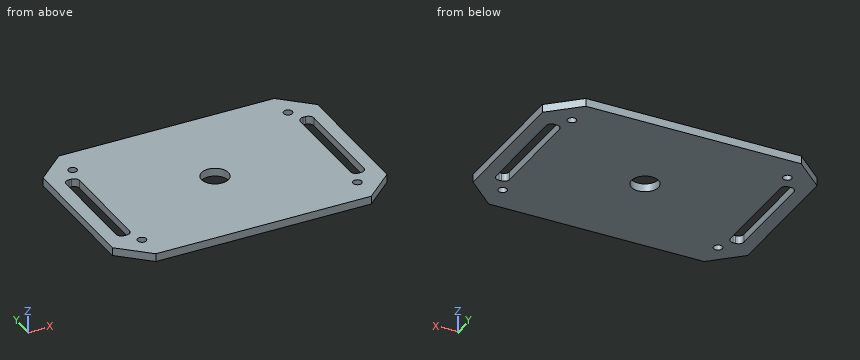
```python
from build123d import *

# Parameters (mm, degrees)
SKETCH1_R           = 1.6
SKETCH1_R_2         = 5
BOSS_EXTRUDE1_DEPTH = 3


with BuildPart() as part:
    # Sketch1 → Boss-Extrude1 (new body)
    with BuildSketch(Plane.XY):
        Polygon((-10.853989547, -33.844947192), (0.146010453, -23.844947192), (80.146010453, -23.844947192), (91.146010453, -33.844947192), (91.146010453, -83.844947192), (80.146010453, -93.844947192), (0.146010453, -93.844947192), (-10.853989547, -83.844947192), align=None)
        with Locations((0.146010453, -33.844947192)):
            Circle(SKETCH1_R, mode=Mode.SUBTRACT)
        with Locations((80.146010453, -33.844947192)):
            Circle(SKETCH1_R, mode=Mode.SUBTRACT)
        with Locations((80.146010453, -83.844947192)):
            Circle(SKETCH1_R, mode=Mode.SUBTRACT)
        with Locations((0.146010453, -83.844947192)):
            Circle(SKETCH1_R, mode=Mode.SUBTRACT)
        with Locations((40.146010453, -58.844947192)):
            Circle(SKETCH1_R_2, mode=Mode.SUBTRACT)
        with BuildLine():
            Line((-3.853989547, -38.844947192), (-2.853989547, -38.844947192))
            ThreePointArc((-2.853989547, -38.844947192), (-1.439775984, -39.430733629), (-0.853989547, -40.844947192))
            Line((-0.853989547, -40.844947192), (-0.853989547, -76.844947192))
            ThreePointArc((-0.853989547, -76.844947192), (-1.439775984, -78.259160754), (-2.853989547, -78.844947192))
            Line((-2.853989547, -78.844947192), (-3.853989547, -78.844947192))
            ThreePointArc((-3.853989547, -78.844947192), (-5.268203109, -78.259160754), (-5.853989547, -76.844947192))
            Line((-5.853989547, -76.844947192), (-5.853989547, -40.844947192))
            ThreePointArc((-5.853989547, -40.844947192), (-5.268203109, -39.430733629), (-3.853989547, -38.844947192))
        make_face(mode=Mode.SUBTRACT)
        with BuildLine():
            Line((84.146010453, -38.844947192), (83.146010453, -38.844947192))
            ThreePointArc((83.146010453, -38.844947192), (81.731796891, -39.430733629), (81.146010453, -40.844947192))
            Line((81.146010453, -40.844947192), (81.146010453, -76.844947192))
            ThreePointArc((81.146010453, -76.844947192), (81.731796891, -78.259160754), (83.146010453, -78.844947192))
            Line((83.146010453, -78.844947192), (84.146010453, -78.844947192))
            ThreePointArc((84.146010453, -78.844947192), (85.560224016, -78.259160754), (86.146010453, -76.844947192))
            Line((86.146010453, -76.844947192), (86.146010453, -40.844947192))
            ThreePointArc((86.146010453, -40.844947192), (85.560224016, -39.430733629), (84.146010453, -38.844947192))
        make_face(mode=Mode.SUBTRACT)
    extrude(amount=BOSS_EXTRUDE1_DEPTH)


solid = part.part
```
The listing builds one solid part. Answer for the finished solid, in the listing's coordinates (mm). Give positions to 0.01 mm unless a question says otherwise; leave off trailing zeros. Order: outer loops, then holes, each group sorted by start corner. A loop starts at its lowest first (then second) coordinate and runs counter-clockwise, first axis right, second up. Notation, with made-up numbers: (57.25, 32) -> (107.25, 32) arc R26 cw to (107.25, 53) -> close; hole circle Ø11 at (40, 33.25). An arc over 180 degrees is marked (long way). Answer as CSV lines item,"result". Start each with the question number.
Q1. Find the intervals of material crossed by L1, parallel to X at y = -48, z = 1.65; L2, parallel to Y at x = 81.5, z = 0.9; L3, parallel to Y at x = 36, z = 1.65, in increasing order.
Q2. A cutting plane is placed at B-B (z = 1.7). Count the separate pieces of the cut face and the enclosed holes in it, then the cut area to 3 significant figures.
Q3. Given pin 1 (1.5 mm diameter, centred on x = 60, y = -50, fed in from -Z); pin 2 (0.5 mm diameter, centred on x = 83.5, z = 2, fed in from -Y), each flat-ended and moving along its own axis, determine where each tip first touches the part or whether it passes through.
Q4. A cutting plane is placed at A-A (y = -75). Determine the outline of the cut face in (x, z).
Results found:
1,L1,"-10.85 to -5.85, -0.85 to 81.15, 86.15 to 91.15"
1,L2,"-92.61 to -84.7, -82.99 to -77.98, -39.71 to -34.7, -32.99 to -25.08"
1,L3,"-93.84 to -61.64, -56.05 to -23.84"
2,separate pieces,"1"
2,enclosed holes,"7"
2,area,"6,420 mm2"
3,pin 1,"z = 0"
3,pin 2,"y = -91.02"
4,outline,"(-10.85, 0) -> (-5.85, 0) -> (-5.85, 3) -> (-10.85, 3) -> close; (-0.85, 0) -> (81.15, 0) -> (81.15, 3) -> (-0.85, 3) -> close; (86.15, 0) -> (91.15, 0) -> (91.15, 3) -> (86.15, 3) -> close"
